```python
from build123d import *

# Parameters (mm, degrees)
F1_DEPTH = 50
F2_R     = 2.5
F3_DEPTH = 12


with BuildPart() as f1:
    # F0 (on Front) → F1 (new body)
    with BuildSketch(Plane.XZ):
        with BuildLine():
            Line((24, -19.5), (24, 19.5))
            Line((24, 19.5), (-24, 19.5))
            Line((-24, 19.5), (-24, -19.5))
            Line((-24, -19.5), (-5, -19.5))
            Line((-5, -19.5), (-5, -12.160254))
            ThreePointArc((-5, -12.160254), (0, 6.5), (5, -12.160254))
            Line((5, -12.160254), (5, -19.5))
            Line((5, -19.5), (24, -19.5))
        make_face()
    extrude(amount=F1_DEPTH)

    # F2 (on face) → F3 (cut)
    with BuildSketch(Plane.XY.offset(19.5)):
        with Locations((-17.5, -42.5)):
            Circle(F2_R)
        with Locations((-17.5, -7.5)):
            Circle(F2_R)
        with Locations((17.5, -7.5)):
            Circle(F2_R)
        with Locations((17.5, -42.5)):
            Circle(F2_R)
    extrude(amount=-F3_DEPTH, mode=Mode.SUBTRACT)


solid = f1.part
```
Geometry: final body of the model. Coordinates: model frame, mm. A direction names the side the tool comes from. Round coordinates to 2 decimals unless told otherwise and drop trailing zeros. Order: outer loops, then holes, each group sorted by start corner. A loop starts at its lowest first (then second) coordinate and runs counter-clockwise, first axis right, second up. Notation, with made-up numbers: M -3,63 L 7,63 A20 cw 7,84 Z; hole C 59.25,60 d11. An arc over 180 degrees is marked long. Use one line per item in the form item = value. Start each with the question number.
Q1. Cut plane B-B (y = -42.5). Return loops of the section in (x, z), and give its area (3 significant figures).
Q2. Material intervals for line 1 (Y direction, x = -17.5, z = 13.25); line 2 (Y direction, x = -17, z = 14); line 3 (X direction, y = -42, z = 13), sorted ascending. Write a range as [from, to].
Q3. Mould query, pull axis X, two halves, no side actions, for faces 4 (the face through (0, -50, 9)), 5 (the face through (24, -25, 0)), 6 (the face through (17, -42, 7.5)). Classes: +X half, -X half, draft (parallel to the pull), parting line (faces both ways), or undercut.
Q4. Cut plane D-D (z = 17). Return loops of the section in (x, y).
Q5. Pin query (flat end, axial travel): pin 1 Ø1.5 at (x, y) = (-18.5, -41.5) entering from +Z; pin 2 Ø8 at (x, z) = (2, -7.5) entering from -Y. Return the tip coordinate at first contact, or that it passes through.
Q6. Cut plane A-A (z = -3.5). Return loops of the section in (x, y).
Q7. Cut plane C-C (x = 17.5). Return loops of the section in (y, z).
Q8. Access query for faces 1 (the face through (15.5, -44, 13.6)), 2 (the face through (-5, -25, -16)), 3 (the face through (-15, -25, -19.5)). Directions: +Z, -Z, +X, -X, +Y, -Y. A direction counts if a zero-diameter tool reaches every point of the face in a straight line with its end or side. Return the directions, or none.
Geometry results:
q1.outline = M -24,-19.5 L -5,-19.5 L -5,-12.16 A10 cw long 5,-12.16 L 5,-19.5 L 24,-19.5 L 24,19.5 L 20,19.5 L 20,7.5 L 15,7.5 L 15,19.5 L -15,19.5 L -15,7.5 L -20,7.5 L -20,19.5 L -24,19.5 Z
q1.area = 1,370 mm^2
q2.line_1 = [-50, -45], [-40, -10], [-5, 0]
q2.line_2 = [-50, -44.95], [-40.05, -9.95], [-5.05, 0]
q2.line_3 = [-24, -19.95], [-15.05, 15.05], [19.95, 24]
q3.face_4 = draft
q3.face_5 = +X half
q3.face_6 = undercut
q4.outline = M -24,-50 L 24,-50 L 24,0 L -24,0 Z; hole C -17.5,-42.5 d5; hole C -17.5,-7.5 d5; hole C 17.5,-42.5 d5; hole C 17.5,-7.5 d5
q5.pin_1 = 7.5
q5.pin_2 = through
q6.outline = M -24,-50 L -10,-50 L -10,0 L -24,0 Z; M 10,-50 L 24,-50 L 24,0 L 10,0 Z
q7.outline = M -50,-19.5 L 0,-19.5 L 0,19.5 L -5,19.5 L -5,7.5 L -10,7.5 L -10,19.5 L -40,19.5 L -40,7.5 L -45,7.5 L -45,19.5 L -50,19.5 Z
q8.face_1 = +Z
q8.face_2 = -Z, +Y, -Y
q8.face_3 = -Z, +X, -X, +Y, -Y
